For this review, take the finished solid that the model builds, in its own axes (mm). Face numbers are marked on the shaded views. A direction names the side the tool comes from. Give positions to 0.01 mm unless a question says otherwise; leave off trailing zeros. Order: outer loops, then holes, each group sorted by start corner. A loop starts at its lowest first (then second) coordinate and runs counter-clockwise, first axis right, second up. Notation, with made-up numbers: M 19,80 L 54,80 A9 cw 54,88 Z; hole C 11.25,43.5 d9. An arc over 180 degrees is marked long. Answer as CSV lines item,"result". Start each with the question number.
1. Clearance check with flat-ended pins moving along their axes: P1, Ø1.5, axis at x = 37.5, y = 22.5, coming from the +Z side; P2, Ø12, axis at x = 21, y = 22.5, coming from the +Z side; P3, Ø4, axis at y = 35.5, z = -0.5, coming from the -X side. State where each tip first meets the part, or that it passes through.
2. We need section A-A, the plane z = 10. Give the boundary of the cut face in (x, y), and give its area (3 significant figures).
3. Mouldability with a two-part tool opening along X and no side actions: class the marked faces 1, 2 and 3 as pulls with the +X half, pulls with the -X half, needs draft (parallel to the pull), parting line crosses it, or undercut.
4. We need section B-B, the plane y = 23. Give the boundary of the cut face in (x, z), and give its area (3 significant figures).
5. Machinability: for the marked faces 4 and 5, which of the approach directions +Z, -Z, +X, -X, +Y, -Y give a long, thin tool a straight path to every point of the face, cutting with its end or side? Answer none if there is none.
6. For line 1 along Z through (x, y) = (19.5, 26); line 2 along X through (y, z) = (22, 4); line 3 along X through (y, z) = (29, 3), list the stretches that pass through material, from the lowest coordinate up.
7. We need section D-D, the plane z = 21.5. Give the boundary of the cut face in (x, y), and give its area (3 significant figures).
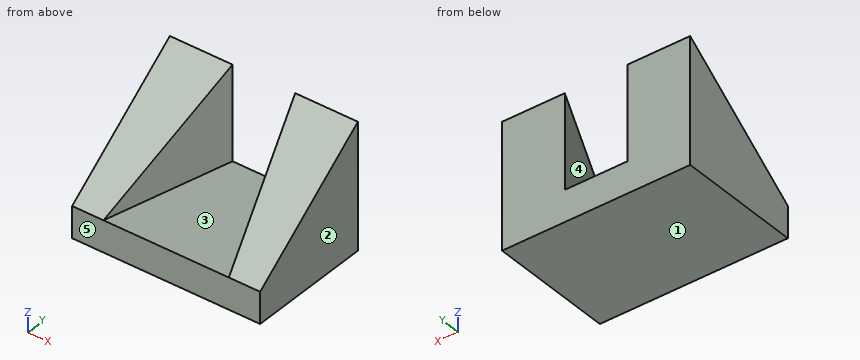
from build123d import *

# Parameters (mm, degrees)
F1_DEPTH   = 10
F2_DEPTH   = 30
F3_SIZE2   = 29.99999
F3_SIZE    = 39.99999
F3_2_SIZE2 = 29.99999
F3_2_SIZE  = 39.99999


# Not quite as in the source:
# - a fillet or chamfer is up to 0.001 mm smaller than in the source, because OpenCascade refuses the exact size


with BuildPart() as f1:
    # F0 (on Top) → F1 (new body)
    with BuildSketch(Plane.XY):
        Polygon((0, 40), (0, 0), (10, 0), (20, 40), align=None)
        Polygon((20, 40), (10, 0), (50, 0), (40, 40), align=None)
        Polygon((40, 40), (50, 0), (60, 0), (60, 40), align=None)
    extrude(amount=-F1_DEPTH)

    # F0 (on Top) → F2 (join)
    with BuildSketch(Plane.XY):
        Polygon((0, 40), (0, 0), (10, 0), (20, 40), align=None)
        Polygon((40, 40), (50, 0), (60, 0), (60, 40), align=None)
    extrude(amount=F2_DEPTH)

    # F3 (size 40 and 30 in the source; OpenCascade refuses exactly that, so slightly less here)
    f3_edges = [f1.edges().sort_by_distance(p)[0] for p in [
        (5, 0, 30),
    ]]
    f3_side = f1.faces().sort_by_distance((7.777778, 22.222222, 30))[0]
    chamfer(f3_edges, length=F3_SIZE, length2=F3_SIZE2, reference=f3_side)

    # F3#2 (size 40 and 30 in the source; OpenCascade refuses exactly that, so slightly less here)
    f3_2_edges = [f1.edges().sort_by_distance(p)[0] for p in [
        (55, 0, 30),
    ]]
    f3_2_side = f1.faces().sort_by_distance((52.222222, 22.222222, 30))[0]
    chamfer(f3_2_edges, length=F3_2_SIZE, length2=F3_2_SIZE2, reference=f3_2_side)


solid = f1.part
Result set:
1,P1,"z = 0"
1,P2,"z = 19.98"
1,P3,"x = 0"
2,outline,"M 0,13.33 L 13.33,13.33 L 20,40 L 0,40 Z; M 40,40 L 46.67,13.33 L 60,13.33 L 60,40 Z"
2,area,"889 mm2"
3,face 1,"needs draft"
3,face 2,"pulls with the +X half"
3,face 3,"undercut"
4,outline,"M 0,-10 L 60,-10 L 60,17.25 L 44.25,17.25 L 44.25,0 L 15.75,0 L 15.75,17.25 L 0,17.25 Z"
4,area,"1,140 mm2"
5,face 4,"+Z, -Y"
5,face 5,"+Z, -Z, +X, -X, -Y"
6,line 1,"-10 to 0"
6,line 2,"0 to 15.5, 44.5 to 60"
6,line 3,"0 to 17.25, 42.75 to 60"
7,outline,"M 0,28.67 L 17.17,28.67 L 20,40 L 0,40 Z; M 40,40 L 42.83,28.67 L 60,28.67 L 60,40 Z"
7,area,"421 mm2"
